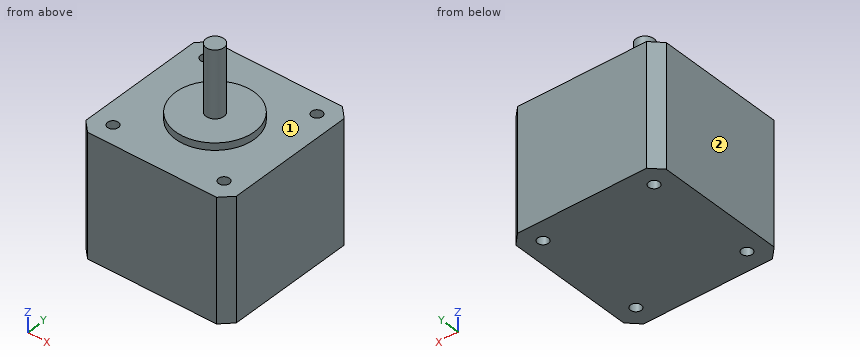
Autodesk Fusion 360 part; units mm, degrees
sketch "Sketch1" plane through (0, 0, 0) normal (0, 0, 1) x (1, 0, 0)
  line L0 (21, 21) -> (-21, 21)
  line L1 (-21, 21) -> (-21, -21)
  line L2 (-21, -21) -> (21, -21)
  line L3 (21, -21) -> (21, 21)
  line L4 (21, 21) -> (-21, -21) construction
  line L5 (-21, 21) -> (21, -21) construction
  circle A0 centre (0, 0) radius 11
  circle A1 centre (0, 0) radius 2.5
  circle A2 centre (-15.5, 15.5) radius 1.5
  circle A3 centre (15.5, 15.5) radius 1.5
  circle A4 centre (15.5, -15.5) radius 1.5
  circle A5 centre (-15.5, -15.5) radius 1.5
  line L6 (-15.5, -15.5) -> (-15.5, 15.5) construction
  line L7 (15.5, 15.5) -> (-15.5, 15.5) construction
  line L8 (15.5, -15.5) -> (15.5, 15.5) construction
  line L9 (-15.5, -15.5) -> (15.5, -15.5) construction
  dimension "d1" = 42
  dimension "d2" = 42
  dimension "d3" = 22
  dimension "d4" = 5
  dimension "d12" = 3
  dimension "d13" = 3
  dimension "d14" = 3
  dimension "d15" = 3
  dimension "d16" = 31
extrude "Extrude1" add sketch "Sketch1" against normal blind 34 contours L0 L1 L2 L3 | A0 | A1
extrude "Extrude2" add sketch "Sketch1" along normal blind 2 contours A0
extrude "Extrude3" add sketch "Sketch1" along normal blind 20.5 contours A1
chamfer "Chamfer1" distance 3 angle 45 4 edges at (21, -21, -17) (-21, -21, -17) (-21, 21, -17) (21, 21, -17)
Geometry check sheet. Reference: the model listing, model coordinates, mm. Face numbers are marked on the shaded views. A direction names the side the tool comes from. Give positions to 0.01 mm unless a question says otherwise; leave off trailing zeros. Order: outer loops, then holes, each group sorted by start corner. A loop starts at its lowest first (then second) coordinate and runs counter-clockwise, first axis right, second up. Notation, with made-up numbers: (-11.5, 71) - (18.5, 71) arc R28 ccw to (18.5, 108) - close; hole circle Ø4 at (61, 46). An arc over 180 degrees is marked (long way). Answer in a Markdown table with one row per item. Add a question column.
Q1. Material ranges on probe 1 along Y at (x, z) = (-15.5, -16); probe 2 along X at (y, z) = (16.5, -32); probe 3 along Z at (x, y) = (-10.5, 9.5), recorded low to high. Write a range as from..to.
Q2. Cross-section at C-C, the plane z = -23.5. Enter the section's corners in (x, y).
Q3. Gauge pin test, flat ends, axial feed: pin 1 (12 mm diameter, centred on x = 15, y = 0, fed in from +Z); pin 2 (5 mm diameter, centred on x = -15.5, y = -15.5, fed in from +Z); pin 3 (2.5 mm diameter, centred on x = -15.5, y = 15.5, fed in from +Z); pin 4 (4 mm diameter, centred on y = 14.5, z = 1, fed in from -X). Record the tip position at first contact, or that the pin passes through.
Q4. Cross-section at A-A, the plane x = -15.5. Enter the section's corners in (y, z), then the cut area to 3 significant figures.
Q5. Cross-section at D-D, the plane x = 0. Enter the section's corners in (y, z), then the cut area to 3 significant figures.
Q6. Tool access check on the marked faces 1 and 2. Record the directions out of +Z, -Z, +X, -X, +Y, -Y that give a thin tool (end or side, any length) a straight path to the whole face; none if there is none.
Check values:
| question | item | result |
|---|---|---|
| 1 | probe 1 | y = -21..-17, -14..14, 17..21 |
| 1 | probe 2 | x = -21..-16.62, -14.38..14.38, 16.62..21 |
| 1 | probe 3 | z = -34..0 |
| 2 | outline | (-21, -18) - (-18, -21) - (18, -21) - (21, -18) - (21, 18) - (18, 21) - (-18, 21) - (-21, 18) - close; hole circle Ø3 at (-15.5, -15.5); hole circle Ø3 at (-15.5, 15.5); hole circle Ø3 at (15.5, -15.5); hole circle Ø3 at (15.5, 15.5) |
| 3 | pin 1 | stops at z = 2 |
| 3 | pin 2 | stops at z = 0 |
| 3 | pin 3 | passes through |
| 3 | pin 4 | stops at x = -21 |
| 4 | outline | (-21, -34) - (-17, -34) - (-17, 0) - (-21, 0) - close; (-14, -34) - (14, -34) - (14, 0) - (-14, 0) - close; (17, -34) - (21, -34) - (21, 0) - (17, 0) - close |
| 4 | area | 1,220 mm^2 |
| 5 | outline | (-21, -34) - (21, -34) - (21, 0) - (11, 0) - (11, 2) - (2.5, 2) - (2.5, 20.5) - (-2.5, 20.5) - (-2.5, 2) - (-11, 2) - (-11, 0) - (-21, 0) - close |
| 5 | area | 1,560 mm^2 |
| 6 | face 1 | +Z |
| 6 | face 2 | +Z, -Z, -X, +Y, -Y |
